from build123d import *

# Parameters (mm, degrees)
SKETCH_1_W          = 20
SKETCH_1_H          = 30
EXTRUDE_1_DEPTH     = 15
CUT_EXTRUDE_1_DEPTH = 10
CUT_EXTRUDE_2_DEPTH = 10


with BuildPart() as part:
    # 草圖1 → 填料-伸長1 (new body)
    with BuildSketch(Plane(origin=(0, 0, 0), x_dir=(1, 0, 0), z_dir=(0, 1, 0))):
        Rectangle(SKETCH_1_W, SKETCH_1_H)
    extrude(amount=EXTRUDE_1_DEPTH)

    # 草圖2 → 除料-伸長1 (cut)
    with BuildSketch(Plane.XY.offset(15)):
        with BuildLine():
            Line((10, 15), (-10, 15))
            ThreePointArc((-10, 15), (0, 5), (10, 15))
        make_face()
    extrude(amount=-CUT_EXTRUDE_1_DEPTH, mode=Mode.SUBTRACT)

    # 草圖3 → 除料-伸長2 (cut)
    with BuildSketch(Plane.XY.offset(5)):
        Polygon((-10, 15), (0, 5), (10, 15), align=None)
    extrude(amount=-CUT_EXTRUDE_2_DEPTH, mode=Mode.SUBTRACT)


solid = part.part
Read the model definition and answer for the solid it produces. Units are mm, in the model's axes. A direction names the side the tool comes from. Coordinates: 2 decimals unless noted, no trailing zeros. Write each loop counter-clockwise with the first axis right and the second up, starting at its lowest first coordinate (ties: lowest second). Pieces come first, ordered by that corner, then holes. Notation, with made-up numbers: (-36, -6.75) -> (19, -6.75) arc R25 cw to (19, 12.25) -> close; hole circle Ø6 at (19.5, 32.5). An arc over 180 degrees is marked (long way). Return JSON: item names as keys, results as strings.
(1) For a pull along Z with two mould halves and no side action, classify faces 3 (the flat face through (-6, 9, 5)), 4 (the flat face through (-5, 10, 0)), 5 (the flat face through (0, 7, -15)) as pulls with the +Z half, pulls with the -Z half, needs draft (parallel to the pull), parting line crosses it, or undercut.
Answers below:
{"face 3": "pulls with the +Z half", "face 4": "needs draft", "face 5": "pulls with the -Z half"}
(2) Each of these flat-tipped pins is pushed along its axis until it touches: P1, Ø2, axis at x = 1, y = 11.5, coming from the +Z side; P2, Ø3, axis at x = 6, y = 11, coming from the +Z side; P3, Ø8, axis at x = -1, y = 8, coming from the +Z side. Where does it stop, or does it pass through?
Answers below:
{"P1": "z = -5", "P2": "z = 5", "P3": "z = 15"}
(3) Consider line 1 along Z through (x, y) = (-0.25, 5.75); line 2 along Z through (x, y) = (1.75, 5.75); line 3 along X through (y, z) = (12, -3.75). Determine where each line is inside the solid, lowest interval first. Write a range as from..to.
Answers below:
{"line 1": "-15..-5", "line 2": "-15..5", "line 3": "-10..-7, 7..10"}
(4) The part is cut by section A-A on z = -2.75. Give the vertices of the cut face in (x, y).
Answers below:
{"outline": "(-10, 0) -> (10, 0) -> (10, 15) -> (0, 5) -> (-10, 15) -> close"}
(5) Which of the six approach directions +Z, -Z, +X, -X, +Y, -Y give full straight-line access (tool end or side, diameter ignored) to faces 1 (the flat face through (0, 11, -5)), 2 (the flat face through (10, 7, 0))?
Answers below:
{"face 1": "+Z, +Y", "face 2": "+Z, -Z, +X, +Y, -Y"}
(6) The part is cut by section C-C on y = 11.5. Give the vertices of the cut face in (x, z).
Answers below:
{"outline": "(-10, -15) -> (10, -15) -> (10, 15) -> (9.37, 15) -> (9.37, 5) -> (6.5, 5) -> (6.5, -5) -> (-6.5, -5) -> (-6.5, 5) -> (-9.37, 5) -> (-9.37, 15) -> (-10, 15) -> close"}
(7) The part is cut by section D-D on x = -4.25. Give the vertices of the cut face in (y, z), then the cut area to 3 significant figures.
Answers below:
{"outline": "(0, -15) -> (15, -15) -> (15, -5) -> (9.25, -5) -> (9.25, 5) -> (5.95, 5) -> (5.95, 15) -> (0, 15) -> close", "area": "302 mm^2"}
(8) The part is cut by section B-B on x = 8.5. Give the vertices of the cut face in (y, z), then the cut area to 3 significant figures.
Answers below:
{"outline": "(0, -15) -> (15, -15) -> (15, -5) -> (13.5, -5) -> (13.5, 5) -> (9.73, 5) -> (9.73, 15) -> (0, 15) -> close", "area": "382 mm^2"}
